Read the model definition and answer for the solid it produces. Units are mm, in the model's axes. Coordinates: 2 decimals unless noted, no trailing zeros. Loops run counter-clockwise (first coordinate to the right, second up) from the corner with the lowest first, then second, coordinate; pieces in that order, holes last.
from build123d import *

# Parameters (mm, degrees)
BOSS_EXTRUDE1_DEPTH                             = 3.175
CSK_FOR_M3_FLAT_HEAD_MACHINE_SCREW1_D           = 3.4
CSK_FOR_M3_FLAT_HEAD_MACHINE_SCREW1_DEPTH       = 7.62
CSK_FOR_M3_FLAT_HEAD_MACHINE_SCREW1_CSINK_D     = 6.3
CSK_FOR_M3_FLAT_HEAD_MACHINE_SCREW1_CSINK_ANGLE = 90
CSK_FOR_M3_FLAT_HEAD_MACHINE_SCREW1_TIP         = 1.021463052
CSK_FOR_M3_FLAT_HEAD_MACHINE_SCREW2_D           = 3.4
CSK_FOR_M3_FLAT_HEAD_MACHINE_SCREW2_DEPTH       = 7.62
CSK_FOR_M3_FLAT_HEAD_MACHINE_SCREW2_CSINK_D     = 6.3
CSK_FOR_M3_FLAT_HEAD_MACHINE_SCREW2_CSINK_ANGLE = 90
CSK_FOR_M3_FLAT_HEAD_MACHINE_SCREW2_TIP         = 1.021463052


with BuildPart() as part:
    # Sketch1 → Boss-Extrude1 (new body)
    with BuildSketch(Plane(origin=(0, 0, 0), x_dir=(0, 0, -1), z_dir=(1, 0, 0))):
        with BuildLine():
            Line((-11.281730167, 3.571875), (11.281730167, 3.571875))
            ThreePointArc((11.281730167, 3.571875), (14.853605167, 0), (11.281730167, -3.571875))
            Line((11.281730167, -3.571875), (-11.281730167, -3.571875))
            ThreePointArc((-11.281730167, -3.571875), (-14.853605167, 0), (-11.281730167, 3.571875))
        make_face()
    extrude(amount=BOSS_EXTRUDE1_DEPTH)

    # CSK for M3 Flat Head Machine Screw1
    with Locations(Plane.ZY):
        with Locations((-11.281730167, 0)):
            CounterSinkHole(CSK_FOR_M3_FLAT_HEAD_MACHINE_SCREW1_D / 2, CSK_FOR_M3_FLAT_HEAD_MACHINE_SCREW1_CSINK_D / 2, depth=CSK_FOR_M3_FLAT_HEAD_MACHINE_SCREW1_DEPTH, counter_sink_angle=CSK_FOR_M3_FLAT_HEAD_MACHINE_SCREW1_CSINK_ANGLE)
            with Locations((0, 0, -(CSK_FOR_M3_FLAT_HEAD_MACHINE_SCREW1_DEPTH + CSK_FOR_M3_FLAT_HEAD_MACHINE_SCREW1_TIP / 2))):  # 118° drill point
                Cone(0, CSK_FOR_M3_FLAT_HEAD_MACHINE_SCREW1_D / 2, CSK_FOR_M3_FLAT_HEAD_MACHINE_SCREW1_TIP, mode=Mode.SUBTRACT)

    # CSK for M3 Flat Head Machine Screw2
    with Locations(Plane(origin=(3.175, 0, 0), x_dir=(0, 0, -1), z_dir=(1, 0, 0))):
        with Locations((-11.281730167, 0)):
            CounterSinkHole(CSK_FOR_M3_FLAT_HEAD_MACHINE_SCREW2_D / 2, CSK_FOR_M3_FLAT_HEAD_MACHINE_SCREW2_CSINK_D / 2, depth=CSK_FOR_M3_FLAT_HEAD_MACHINE_SCREW2_DEPTH, counter_sink_angle=CSK_FOR_M3_FLAT_HEAD_MACHINE_SCREW2_CSINK_ANGLE)
            with Locations((0, 0, -(CSK_FOR_M3_FLAT_HEAD_MACHINE_SCREW2_DEPTH + CSK_FOR_M3_FLAT_HEAD_MACHINE_SCREW2_TIP / 2))):  # 118° drill point
                Cone(0, CSK_FOR_M3_FLAT_HEAD_MACHINE_SCREW2_D / 2, CSK_FOR_M3_FLAT_HEAD_MACHINE_SCREW2_TIP, mode=Mode.SUBTRACT)


solid = part.part
Q1. A cutting plane is placed at B-B (x = 2.8). Give the vertices of the cut face in (y, z) (3 decimals).
Findings below:
outline: (-3.572, -11.282) arc R3.572 ccw to (3.572, -11.282) - (3.572, 11.282) arc R3.572 ccw to (-3.572, 11.282) - close; hole circle Ø5.55 at (0, 11.282); hole circle Ø3.4 at (0, -11.282)
Q2. A flat-ended cylindrical pin translates along its axis: pin 1 Ø2.5 at (y, z) = (0, -11.28) entering from -X. Find the tip coordinate at first contact, or state that the pin passes through.
Findings below:
pin 1: passes through
Q3. A cutting plane is placed at C-C (x = 0.8). Give the vertices of the cut face in (y, z), then the cut area to 3 significant figures.
Findings below:
outline: (-3.57, -11.28) arc R3.57 ccw to (3.57, -11.28) - (3.57, 11.28) arc R3.57 ccw to (-3.57, 11.28) - close; hole circle Ø4.7 at (0, -11.28); hole circle Ø3.4 at (0, 11.28)
area: 175 mm2
Q4. Straight lines are drawn through the part: probe 1 along Z at (x, y) = (0.5, 0); probe 2 along Z at (x, y) = (0.75, -1); probe 3 along Y at (x, z) = (1.45, 12.25). For each, find the intervals that lie inside material, in ascending order.
Findings below:
probe 1: z = -14.85 to -13.93, -8.63 to 9.58, 12.98 to 14.85
probe 2: z = -14.71 to -13.46, -9.1 to 9.91, 12.66 to 14.71
probe 3: y = -3.44 to -1.4, 1.4 to 3.44
Q5. Determine the mould class of faces 1 (the face through (0.85, 0.075, 9.583)), 2 (the face through (3.175, 0, -4)), 3 (the face through (1.565, 0.079, -14.853)), 4 (the face through (2.325, 0.075, -9.583)) for opening direction Y: +Y half, -Y half, draft (parallel to the pull), parting line (faces both ways), or undercut.
Findings below:
face 1: undercut
face 2: draft
face 3: parting line
face 4: undercut
Q6. A cutting plane is placed at A-A (y = 0). Give the vertices of the cut face in (x, z) (3 decimals), then the cut area to 3 significant figures.
Findings below:
outline: (0, -14.854) - (3.175, -14.854) - (3.175, -12.982) - (1.45, -12.982) - (0, -14.432) - close; (0, -8.132) - (1.45, -9.582) - (3.175, -9.582) - (3.175, 8.132) - (1.725, 9.582) - (0, 9.582) - close; (0, 12.982) - (1.725, 12.982) - (3.175, 14.432) - (3.175, 14.854) - (0, 14.854) - close
area: 68.5 mm2
